Can you work these out from the drawing? Everything is in mm from the part's minimum corner. Coordinates: 2 decimals unless noted, no trailing zeros. Write each loop counter-clockwise with the first axis right and the second up, starting at its lowest first coordinate (ties: lowest second). Pieces come first, ordered by that corner, then holes.
(1) Please list where these lines run through material, in increasing order: probe 1 along X at (y, z) = (18.25, 0.8) (1 decimal); probe 2 along X at (y, z) = (20.5, 0.5) (1 decimal); probe 3 along Y at (x, z) = (1.75, 0.6) (1 decimal).
(2) Imagine slicing it at B-B, the plane x = 17.75. List the corners of the cut face in (y, z) for me, plus the area to 3 significant figures.
(3) Imagine slicing it at C-C, the plane z = 1.05. List the corners of the cut face in (x, y) for me.
(4) For pin 1 Ø5 at (x, y) = (3.05, 19.24) entering from -Z, with a flat end and sliding along its axis, tell me the tip position at first contact or that it passes through.
(5) Thinking about a two-plate mould opening in X: for the marked faces 1 and 2, which applies, released by +X, released by -X, zero draft, split by the parting line, or undercut?
(6) Imagine slicing it at D-D, the plane y = 7.5. List the corners of the cut face in (x, z) for me (1 decimal).
(7) Imagine slicing it at A-A, the plane y = 3. List the corners of the cut face in (x, z) for me.
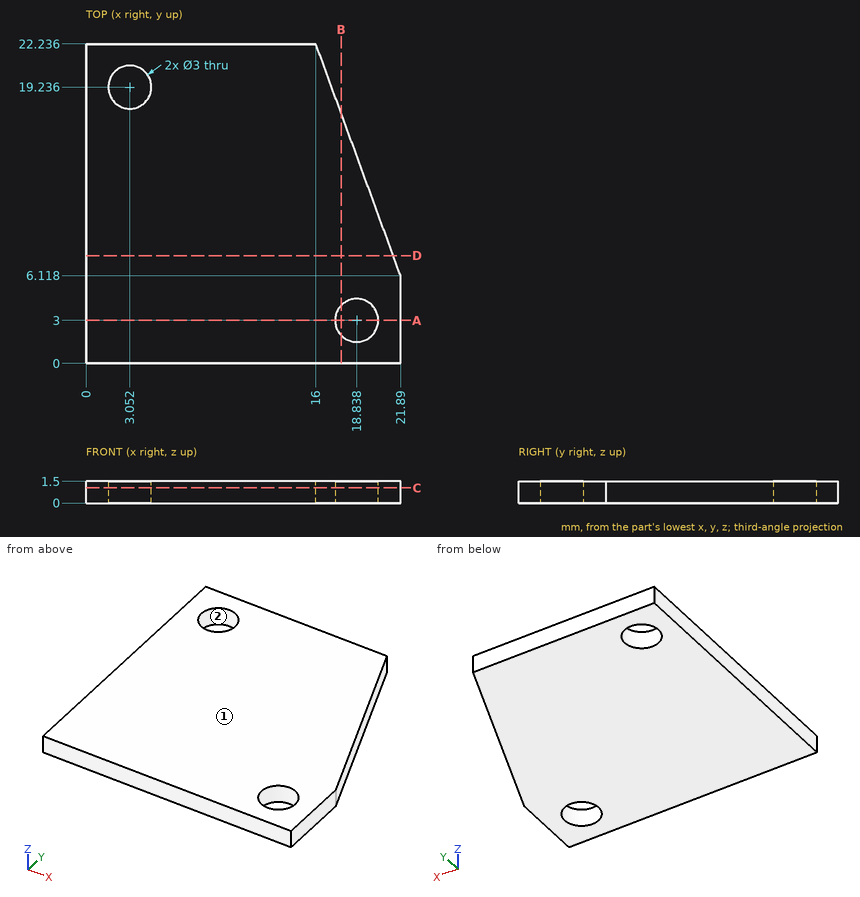
Recorded:
1. probe 1: x = 0 to 1.9, 4.2 to 17.5
1. probe 2: x = 0 to 2.2, 3.9 to 16.6
1. probe 3: y = 0 to 18.5, 20 to 22.2
2. outline: (0, 0) - (1.97, 0) - (1.97, 1.5) - (0, 1.5) - close; (4.03, 0) - (17.45, 0) - (17.45, 1.5) - (4.03, 1.5) - close
2. area: 23.1 mm2
3. outline: (0, 0) - (21.89, 0) - (21.89, 6.12) - (16, 22.24) - (0, 22.24) - close; hole circle Ø3 at (3.05, 19.24); hole circle Ø3 at (18.84, 3)
4. pin 1: stops at z = 0
5. face 1: zero draft
5. face 2: undercut
6. outline: (0, 0) - (21.4, 0) - (21.4, 1.5) - (0, 1.5) - close
7. outline: (0, 0) - (17.34, 0) - (17.34, 1.5) - (0, 1.5) - close; (20.34, 0) - (21.89, 0) - (21.89, 1.5) - (20.34, 1.5) - close
